```python
from build123d import *

# Parameters (mm, degrees)
F0_W         = 6
F0_H         = 11
F0_R         = 1.5
F1_DEPTH     = 3
F2_DEPTH     = 9
F3_W         = 6
F3_H         = 3.2
F4_DEPTH     = 15
F5_W         = 5
F5_H         = 6
F6_DEPTH     = 1
F7_T1_DEPTH  = 31
F8_R         = 3
F9_R         = 1
F10_T1_DEPTH = 3
F11_R        = 2


# Not quite as in the source:
# - a fillet or chamfer that OpenCascade refuses, or shapes differently, is made with other operations: its cross-section is extruded or revolved along the edge and cut away or added


with BuildPart() as f1:
    # F0 (on Top) → F1 (new body)
    with BuildSketch(Plane.XY):
        with Locations((-92, 0)):
            Rectangle(F0_W, F0_H)
        Polygon((-89, -5.5), (95, -5.5), (95, -3), (115, -3), (115, 3), (95, 3), (95, 5.5), (-89, 5.5), align=None)
        Circle(F0_R, mode=Mode.SUBTRACT)
    extrude(amount=F1_DEPTH)

    # F0 (on Top) → F2 (join)
    with BuildSketch(Plane.XY):
        with Locations((-92, 0)):
            Rectangle(F0_W, F0_H)
    extrude(amount=F2_DEPTH)

    # F3 (on face) → F4 (cut, symmetric)
    with BuildSketch(Plane(origin=(-95, 0, 0), x_dir=(0, -1, 0), z_dir=(-1, 0, 0))):
        with Locations((0, 4.6)):
            Rectangle(F3_W, F3_H)
    extrude(amount=F4_DEPTH, both=True, mode=Mode.SUBTRACT)

    # F5 (on face) → F6 (join)
    with BuildSketch(Plane.XY.offset(3)):
        with Locations((107.5, 0)):
            Rectangle(F5_W, F5_H)
    extrude(amount=F6_DEPTH)

    # F7: fillet of radius 13 on 1 edges, made by hand

    # F7_s2 → F7_t1 (cut)
    with BuildSketch(Plane.XZ.offset(-15.5)):
        with BuildLine():
            ThreePointArc((105, 4), (107.5495097568, 3.747548784), (110, 3))
            Line((110, 3), (110, 4))
            Line((110, 4), (105, 4))
        make_face()
    extrude(amount=F7_T1_DEPTH, mode=Mode.SUBTRACT)

    # F8
    f8_edges = [f1.edges().sort_by_distance(p)[0] for p in [
        (-89, -4.25, 3),
        (-89, 4.25, 3),
    ]]
    fillet(f8_edges, radius=F8_R)

    # F9
    f9_edges = [f1.edges().sort_by_distance(p)[0] for p in [
        (115, 0, 3),
    ]]
    fillet(f9_edges, radius=F9_R)

    # F10: fillet of radius 5 on 2 edges, made by hand

    # F10_s2 → F10_t1 (join)
    with BuildSketch(Plane.XY):
        with BuildLine():
            ThreePointArc((99.3301270189, -3), (96.8301270189, -3.6698729811), (95, -5.5))
            Line((95, -5.5), (95, -3))
            Line((95, -3), (99.3301270189, -3))
        make_face()
        with BuildLine():
            ThreePointArc((99.3301270189, 3), (96.8301270189, 3.6698729811), (95, 5.5))
            Line((95, 5.5), (95, 3))
            Line((95, 3), (99.3301270189, 3))
        make_face()
    extrude(amount=F10_T1_DEPTH)

    # F11
    f11_edges = [f1.edges().sort_by_distance(p)[0] for p in [
        (-92, 5.5, 9),
        (-92, -5.5, 9),
    ]]
    fillet(f11_edges, radius=F11_R)


solid = f1.part
```
Read the model definition and answer for the solid it produces. Units are mm, in the model's axes. A direction names the side the tool comes from. Round coordinates to 2 decimals unless told otherwise and drop trailing zeros. Write each loop counter-clockwise with the first axis right and the second up, starting at its lowest first coordinate (ties: lowest second). Pieces come first, ordered by that corner, then holes. Notation, with made-up numbers: M -13.5,36 L 25.5,36 A18 ccw 25.5,61 Z; hole C 47,75 d2. An arc over 180 degrees is marked long. One line per item, written item: value.
Q1. Find section A-A on x = 89. Write down the section's boundary in (y, z).
Data:
outline: M -5.5,0 L 5.5,0 L 5.5,3 L -5.5,3 Z
Q2. Flat-ended cylindrical pins translate along their axes: pin 1 Ø2 at (x, z) = (107.5, 1.5) entering from +Y; pin 2 Ø1.8 at (x, y) = (0, 0) entering from -Z; pin 3 Ø4.5 at (x, y) = (111.5, 0) entering from +Z; pin 4 Ø4 at (x, y) = (61.5, 1.5) entering from +Z. Find the tip coordinate at first contact, or state that the pin passes through.
Data:
pin 1: y = 3
pin 2: through
pin 3: z = 3.29
pin 4: z = 3
Q3. Straight lines are drawn through the part: line 1 (Y direction, x = 0, z = 1.4); line 2 (Z direction, x = 67.5, y = 3.25); line 3 (X direction, y = -1.25, z = 6.5). For each, find the intervals that lie inside material, in ascending order. Write a range as [from, to].
Data:
line 1: [-5.5, -1.5], [1.5, 5.5]
line 2: [0, 3]
line 3: [-95, -89]
Q4. Which of the six approach directions +Z, -Z, +X, -X, +Y, -Y give full straight-line access (tool end or side, diameter ignored) to faces 1 (the flat face through (-92, 3, 5)), 2 (the flat face through (107, 3, 2)), 3 (the flat face through (112, 0, 3)), 4 (the flat face through (-92, 0, 6.2))?
Data:
face 1: -X
face 2: +Z, -Z, +X, +Y
face 3: +Z, +X, +Y, -Y
face 4: +X, -X
Q5. For a pull along Y with two mould halves and no side action, classify faces 5 (the flat face through (-92, -3, 5)), 6 (the flat face through (1, 5.5, 1)), 7 (the flat face through (107, -3, 2)) as +Y half, -Y half, draft (parallel to the pull), parting line (faces both ways), or undercut.
Data:
face 5: undercut
face 6: +Y half
face 7: -Y half
